Autodesk Inventor part; units mm, degrees
ref_plane "YZ Plane" through (0, 0, 0) normal (1, 0, 0) x (0, 1, 0)
ref_plane "XZ Plane" through (0, 0, 0) normal (0, 1, 0) x (-1, 0, 0)
ref_plane "XY Plane" through (0, 0, 0) normal (0, 0, 1) x (1, 0, 0)
sketch "草圖1" plane through (0, 0, 0) normal (0, 1, 0) x (-1, 0, 0)
  line L0 (25, 0) -> (0, 0)
  line L1 (0, 0) -> (0, -20)
  line L2 (0, -20) -> (25, -20)
  line L3 (25, -20) -> (25, 0)
  line L4 (6.5, -14.5) -> (18.5, -14.5) construction
  line L5 (5.5, -17.5) -> (8.5, -17.5)
  line L6 (8.5, -17.5) -> (8.5, -14.5)
  line L7 (8.5, -14.5) -> (5.5, -14.5)
  line L8 (5.5, -14.5) -> (5.5, -17.5)
  line L9 (9, -4.5) -> (16, -4.5) construction
  line L10 (9, -4.5) -> (6, -4.5)
  line L11 (6, -4.5) -> (6, -1.5)
  line L12 (6, -1.5) -> (9, -1.5)
  line L13 (9, -1.5) -> (9, -4.5)
  line L14 (16, -4.5) -> (19, -4.5)
  line L15 (19, -4.5) -> (19, -1.5)
  line L16 (19, -1.5) -> (16, -1.5)
  line L17 (16, -1.5) -> (16, -4.5)
  line L18 (16.5, -17.5) -> (19.5, -17.5)
  line L19 (19.5, -17.5) -> (19.5, -14.5)
  line L20 (19.5, -14.5) -> (16.5, -14.5)
  line L21 (16.5, -14.5) -> (16.5, -17.5)
  circle A0 centre (4, -9.5) radius 1.5
  circle A1 centre (21, -9.5) radius 1.5
  line L22 (11, -14.5) -> (14, -14.5)
  line L23 (14, -14.5) -> (14, -17.5)
  line L24 (14, -17.5) -> (11, -17.5)
  line L25 (11, -17.5) -> (11, -14.5)
  line L26 (25, -18.5) -> (0, -18.5)
  point P0 (19, 16.3854)
  point P1 (12.5, -17.5)
  point P2 (12.5, -14.5)
  dimension "d0" = 25
  dimension "d1" = 20
  dimension "d2" = 3
  dimension "d3" = 3
  dimension "d4" = 0
  dimension "d5" = 10
  dimension "d6" = 3
  dimension "d7" = 3
  dimension "d8" = 3
  dimension "d9" = 3
  dimension "d10" = 3
  dimension "d11" = 3
  dimension "d12" = 3
  dimension "d13" = 5
  dimension "d14" = 5
  dimension "d15" = 8
  dimension "d16" = 2.5
  dimension "d18" = 7
  dimension "d22" = 5.5
  dimension "d23" = 5.5
  dimension "d24" = 6
  dimension "d25" = 3
  dimension "d26" = 3
  dimension "d27" = 1
extrude "擠出1" add sketch "草圖1" along normal blind 3 contours L3 L26 L1 L0 | L8 L7 L6 L5 | L21 L20 L19 L18
sketch "草圖2" plane through (0, 3, 0) normal (0, 1, 0) x (1, 0, 0)
  line L0 (0, 0) -> (0, 18.5)
  line L1 (-25, 18.5) -> (-25, 0)
  line L2 (-25, 0) -> (0, 0)
  circle A0 centre (-21, 9.5) radius 1.5
  circle A1 centre (-4, 9.5) radius 1.5
  line L3 (-11, 14.5) -> (-14, 14.5)
  line L4 (-14, 14.5) -> (-14, 17.5)
  line L5 (-14, 17.5) -> (-11, 17.5)
  line L6 (-11, 17.5) -> (-11, 14.5)
  line L7 (-9, 1.5) -> (-9, 4.5)
  line L8 (-9, 4.5) -> (-6, 4.5)
  line L9 (-6, 4.5) -> (-6, 1.5)
  line L10 (-6, 1.5) -> (-9, 1.5)
  line L11 (-16, 4.5) -> (-16, 1.5)
  line L12 (-16, 1.5) -> (-19, 1.5)
  line L13 (-19, 1.5) -> (-19, 4.5)
  line L14 (-19, 4.5) -> (-16, 4.5)
  line L15 (0, 18.5) -> (-25, 18.5)
properties part number "motorbase_3"
Here's how the part is built. I have some questions about the finished solid (model axes, mm). A direction names the side the tool comes from. Give positions to 0.01 mm unless a question says otherwise; leave off trailing zeros. Loops run counter-clockwise (first coordinate to the right, second up) from the corner with the lowest first, then second, coordinate; pieces in that order, holes last. Notation, with made-up numbers: M 48,63 L 85,63 A32 cw 85,101 Z; hole C 59.25,48.5 d3. An arc over 180 degrees is marked long. Use one line per item in the form item = value. Start each with the question number.
Q1. I need wall thicknesses on line 1 along X through (y, z) = (2.1, -2); line 2 along Z through (x, y) = (-16.5, 0.9); line 3 along Z through (x, y) = (-21, 1.8). Which ranges of each line are inside material? Lowest first, please.
Q2. If we section it at D-D (x = -4.5): Write out the boundary of the cut face in (y, z), then the cut area to 3 significant figures.
Q3. If we section it at C-C (x = -7.25): Write out the boundary of the cut face in (y, z), then the cut area to 3 significant figures.
Q4. If we section it at A-A (z = -9.5): Write out the boundary of the cut face in (x, y), then the cut area to 3 significant figures.
Q5. Thinking about a two-plate mould opening in X: for faces 3 (the flat face through (-14, 1, -16)), 4 (the flat face through (-13, 1, -18.5)), 5 (the flat face through (-12, 1, -14.5)), 6 (the flat face through (-25, 1, -9)), which applies, +X half, -X half, draft (parallel to the pull), parting line (faces both ways), or undercut?
Q6. Will this pin go through, and if not, where does the flat tip stop? pin 1 Ø0.9 at (y, z) = (1.5, -15.5) entering from +X.
Q7. Which directions (+Z, -Z, +X, -X, +Y, -Y) give clear straight access to the entire face, cutting with the end or side of a thin tool? Please do faces 1 (the flat face through (-12, 3, -9)), 2 (the flat face through (-17, 1, -4.5)).
Q8. If we section it at B-B (y = 0.6): Write out the boundary of the cut face in (x, z), then the cut area to 3 significant figures.
Taken from the geometry:
q1.line_1 = -25 to -19, -16 to -9, -6 to 0
q1.line_2 = -18.5 to -4.5, -1.5 to 0
q1.line_3 = -18.5 to -11, -8 to 0
q2.outline = M 0,-18.5 L 3,-18.5 L 3,-10.91 L 0,-10.91 Z; M 0,-8.09 L 3,-8.09 L 3,0 L 0,0 Z
q2.area = 47.0 mm^2
q3.outline = M 0,-18.5 L 3,-18.5 L 3,-4.5 L 0,-4.5 Z; M 0,-1.5 L 3,-1.5 L 3,0 L 0,0 Z
q3.area = 46.5 mm^2
q4.outline = M -25,0 L -22.5,0 L -22.5,3 L -25,3 Z; M -19.5,0 L -5.5,0 L -5.5,3 L -19.5,3 Z; M -2.5,0 L 0,0 L 0,3 L -2.5,3 Z
q4.area = 57.0 mm^2
q5.face_3 = undercut
q5.face_4 = draft
q5.face_5 = undercut
q5.face_6 = -X half
q6.pin_1 = 0
q7.face_1 = +Z, -Z, +X, -X, +Y
q7.face_2 = +Y, -Y
q8.outline = M -25,-18.5 L 0,-18.5 L 0,0 L -25,0 Z; hole C -21,-9.5 d3; hole M -19,-4.5 L -16,-4.5 L -16,-1.5 L -19,-1.5 Z; hole M -14,-17.5 L -11,-17.5 L -11,-14.5 L -14,-14.5 Z; hole M -9,-4.5 L -6,-4.5 L -6,-1.5 L -9,-1.5 Z; hole C -4,-9.5 d3
q8.area = 421 mm^2
